Source: CAD feature listing. Evaluate the final solid. Frame: model axes, mm. Face numbers are marked on the shaded views. A direction names the side the tool comes from. Coordinates: 2 decimals unless noted, no trailing zeros. Order: outer loops, then holes, each group sorted by start corner. A loop starts at its lowest first (then second) coordinate and runs counter-clockwise, first axis right, second up.
Item 1: Mould query, pull axis X, two halves, no side actions, for the marked faces 6, 7 and 8. Classes: released by +X, released by -X, zero draft, split by the parting line, or undercut.
Item 2: Ray query, line 1 (Y direction, x = 4.5, z = -4); line 2 (X direction, y = -34.5, z = -3); line 3 (Z direction, x = 7, y = -7.5). Return the intervals inside material, ascending.
Item 3: Section B-B on y = -4.5. State how many separate pieces and enclosed holes the cut face has, then the cut area to 3 significant figures.
Item 4: Section A-A on z = 0. Return the cut outline in (x, y).
Item 5: Reachability of the marked faces 1, 2, 3, 4 and 5 from +Z, -Z, +X, -X, +Y, -Y: full face, straight path, thin tool, end or side. Return the list, or none.
Item 6: Section D-D on z = 12. Return the cut outline in (x, y).
Item 7: Contact query for flat-ended pins moving along their axis: P1, Ø5, axis at y = -12, z = 13.5, coming from the -X side; P2, Ø10, axis at y = -29, z = 9, coming from the -X side; P3, Ø10, axis at x = 33.5, y = -24.5, coming from the +Z side; P4, Ø3, axis at x = 4.5, y = -34.5, coming from the +Z side. Output: stop coordinate, or through.
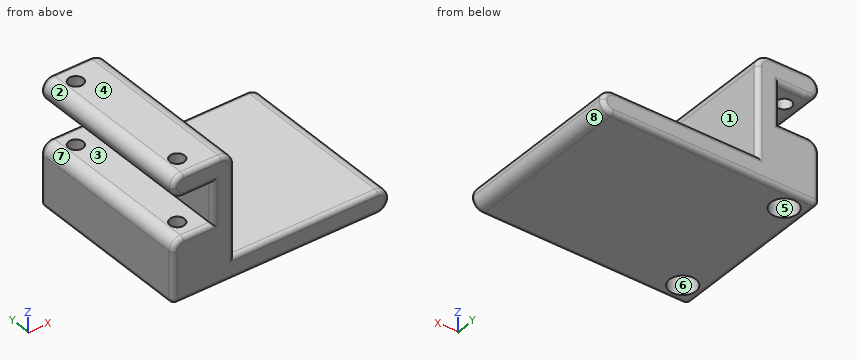
Autodesk Inventor part; units mm, degrees
ref_plane "YZ Plane" through (0, 0, 0) normal (1, 0, 0) x (0, 1, 0)
ref_plane "XZ Plane" through (0, 0, 0) normal (0, 1, 0) x (-1, 0, 0)
ref_plane "XY Plane" through (0, 0, 0) normal (0, 0, 1) x (1, 0, 0)
sketch "スケッチ1" plane through (0, 0, 0) normal (0, 0, 1) x (1, 0, 0)
  line L0 (0, 0) -> (49, 0)
  line L1 (49, 0) -> (49, -39)
  line L2 (49, -39) -> (0, -39)
  line L3 (0, -39) -> (0, 0)
  dimension "d2" = 39
  dimension "d3" = 49
extrude "押し出し1" add sketch "スケッチ1" along normal blind 5
sketch "スケッチ2" plane through (0, 0, 5) normal (0, 0, 1) x (1, 0, 0)
  line L0 (49, 0) -> (0, 0)
  line L1 (9, 0) -> (14, 0)
  line L2 (14, 0) -> (14, -39)
  line L3 (14, -39) -> (9, -39)
  line L4 (9, -39) -> (9, 0)
  line L5 (0, 0) -> (0, -39)
  dimension "d4" = 5
  dimension "d5" = 39
  dimension "d6" = 9
extrude "押し出し2" add sketch "スケッチ2" along normal blind 9
sketch "スケッチ3" plane through (0, 0, 14) normal (0, 0, 1) x (1, 0, 0)
  line L0 (0, -39) -> (9, -39)
  line L1 (14, 0) -> (0, 0)
  line L2 (0, 0) -> (0, -39)
  line L3 (0, -39) -> (14, -39)
  line L4 (14, -39) -> (14, 0)
  point P0 (0, 0)
extrude "押し出し3" add sketch "スケッチ3" along normal blind 5
sketch "スケッチ4" plane through (0, 0, 0) normal (0, 0, -1) x (-1, 0, 0)
  line L0 (-49, 0) -> (-14, 0)
  line L1 (0, -39) -> (-49, -39)
  line L2 (-49, 0) -> (0, 0)
  line L3 (0, 0) -> (0, -39)
  line L4 (0, -39) -> (-49, -39)
  line L5 (-49, -39) -> (-49, 0)
  point P0 (0, 0)
extrude "押し出し4" add sketch "スケッチ4" along normal blind 9
sketch "スケッチ5" plane through (0, 0, 5) normal (0, 0, 1) x (1, 0, 0)
  line L0 (49, 0) -> (14, 0)
  line L1 (14, 0) -> (49, 0)
  line L2 (49, 0) -> (49, -39)
  line L3 (49, -39) -> (14, -39)
  line L4 (14, -39) -> (14, 0)
  point P0 (0, 0)
extrude "押し出し5" cut sketch "スケッチ5" against normal blind 9
fillet "フィレット1" radius 2.5 2 edges at (49, -19.5, -4) (49, -19.5, -9)
fillet "フィレット2" radius 2.5 3 edges at (0, -19.5, 19) (0, -19.5, 14) (0, -19.5, 5)
sketch "スケッチ6" plane through (0, 0, -9) normal (0, 0, -1) x (-1, 0, 0)
  line L0 (0, 0) -> (-46.5, 0)
  line L1 (-46.5, -39) -> (0, -39)
  line L2 (0, -39) -> (0, 0)
  point P0 (-4.5, -4.5)
  point P1 (-4.5, -34.5)
  dimension "d17" = 4.5
  dimension "d18" = 4.5
  dimension "d19" = 4.5
  dimension "d20" = 4.5
hole "穴1" at (4.5, -4.5, -9) at (4.5, -34.5, -9) direction (0, 0, 1) diameter 3.3 end through all counterbore diameter 6 counterbore depth 8
fillet "フィレット5" radius 1 23 edges at (48.2678, 0, -4.7322) (30.2501, 0, -4) (23.25, 0, -9) (0.7322, 0, 4.2678) (5.7499, 0, 5) (0, 0, -3.2499) (9, 0, 9.5) (14, 0, 7.5) (0.7322, 0, 18.2678) (5.75, 0, 14) (8.25, 0, 19) (0, -19.5, -9) (48.2678, -39, -4.7322) (30.2501, -39, -4) (23.2501, -39, -9) (9, -39, 9.5) (0.7322, -39, 18.2678) (8.25, -39, 19) (5.75, -39, 14) (5.75, -39, 5) (0, -39, -3.25) (0.7322, -39, 4.2678) (14, -39, 7.5)
fillet "フィレット6" radius 3 3 edges at (13.7071, -0.2929, 18.7071) (13.7071, -38.7071, 18.7071) (14, -19.5, 19)
properties part number "ハンド3D_L" material "ABS プラスチック"
Answer list:
1. face 6: undercut
1. face 7: released by -X
1. face 8: released by +X
2. line 1: y = -39 to -37.5, -31.5 to -7.5, -1.5 to 0
2. line 2: x = 0 to 1.5, 7.5 to 14
2. line 3: z = -9 to 5, 14 to 19
3. separate pieces: 3
3. enclosed holes: 0
3. area: 393 mm2
4. outline: (0, -38) arc R1 ccw to (1, -39) - (13, -39) arc R1 ccw to (14, -38) - (14, -1) arc R1 ccw to (13, 0) - (1, 0) arc R1 ccw to (0, -1) - close; hole circle Ø3.3 at (4.5, -34.5); hole circle Ø3.3 at (4.5, -4.5)
5. face 1: +Z, +X, +Y, -Y
5. face 2: +Z, -X, +Y, -Y
5. face 3: -X, +Y, -Y
5. face 4: +Z, +X, -X, +Y, -Y
5. face 5: -Z
6. outline: (9, -38) arc R1 ccw to (10, -39) - (13, -39) arc R1 ccw to (14, -38) - (14, -1) arc R1 ccw to (13, 0) - (10, 0) arc R1 ccw to (9, -1) - close
7. P1: stops at x = 0.05
7. P2: stops at x = 0.5
7. P3: stops at z = -4
7. P4: passes through
